Could you check a few things on this drawing? It's one solid part, dimensions in mm from its lowest x, y, z. Give positions to 0.01 mm unless a question says otherwise; leave off trailing zeros. Order: outer loops, then holes, each group sorted by start corner. A loop starts at its lowest first (then second) coordinate and runs counter-clockwise, first axis right, second up. Notation, with made-up numbers: (11.25, 9) -> (48.25, 9) arc R28 cw to (48.25, 32) -> close; hole circle Ø2 at (21.5, 51.5). An arc over 180 degrees is marked (long way). Answer as a JSON object with one key per item and string values.
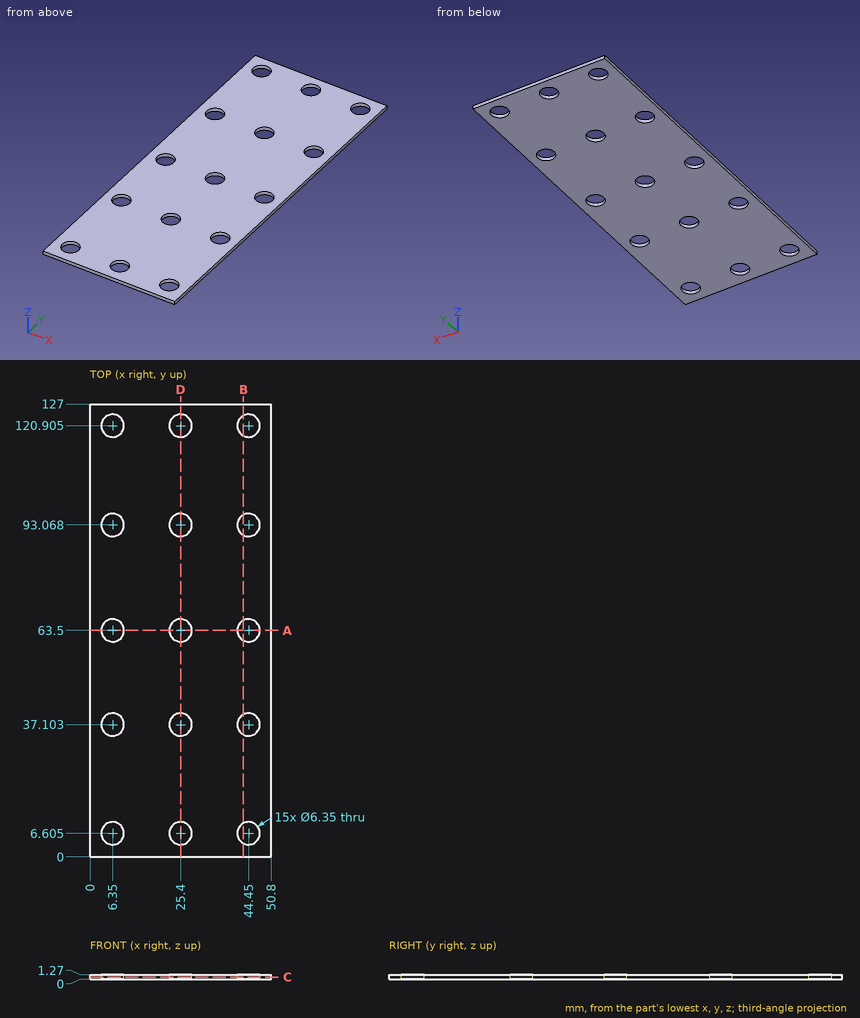
1. Will this pin go through, and if not, where does the flat tip stop? pin 1 Ø10 at (x, y) = (25.4, 120.91) entering from -Z.
Worked answers:
{"pin 1": "z = 0"}
2. If we section it at C-C on z = 0.6: Count the separate pieces of the cut face and the enclosed holes in it, then the cut area to 3 significant figures.
Worked answers:
{"separate pieces": "1", "enclosed holes": "15", "area": "5,980 mm²"}
3. Please list where these lines run through material, in increasing order: L1, parallel to X at y = 63.5, z = 0.4 (1 decimal); L2, parallel to Y at x = 44.45, z = 0.55 (1 decimal); L3, parallel to X at y = 91, z = 1.1.
Worked answers:
{"L1": "0 to 3.2, 9.5 to 22.2, 28.6 to 41.3, 47.6 to 50.8", "L2": "0 to 3.4, 9.8 to 33.9, 40.3 to 60.3, 66.7 to 89.9, 96.2 to 117.7, 124.1 to 127", "L3": "0 to 3.94, 8.76 to 22.99, 27.81 to 42.04, 46.86 to 50.8"}
4. If we section it at A-A on y = 63.5: Please give me the cut outline in (x, z) (1 decimal).
Worked answers:
{"outline": "(0, 0) -> (3.2, 0) -> (3.2, 1.3) -> (0, 1.3) -> close; (9.5, 0) -> (22.2, 0) -> (22.2, 1.3) -> (9.5, 1.3) -> close; (28.6, 0) -> (41.3, 0) -> (41.3, 1.3) -> (28.6, 1.3) -> close; (47.6, 0) -> (50.8, 0) -> (50.8, 1.3) -> (47.6, 1.3) -> close"}
5. If we section it at B-B on x = 43: Please give me the cut outline in (y, z) (1 decimal).
Worked answers:
{"outline": "(0, 0) -> (3.8, 0) -> (3.8, 1.3) -> (0, 1.3) -> close; (9.4, 0) -> (34.3, 0) -> (34.3, 1.3) -> (9.4, 1.3) -> close; (39.9, 0) -> (60.7, 0) -> (60.7, 1.3) -> (39.9, 1.3) -> close; (66.3, 0) -> (90.2, 0) -> (90.2, 1.3) -> (66.3, 1.3) -> close; (95.9, 0) -> (118.1, 0) -> (118.1, 1.3) -> (95.9, 1.3) -> close; (123.7, 0) -> (127, 0) -> (127, 1.3) -> (123.7, 1.3) -> close"}
6. If we section it at D-D on x = 25.4: Please give me the cut outline in (y, z) (1 decimal), then the cut area to 3 significant figures.
Worked answers:
{"outline": "(0, 0) -> (3.4, 0) -> (3.4, 1.3) -> (0, 1.3) -> close; (9.8, 0) -> (33.9, 0) -> (33.9, 1.3) -> (9.8, 1.3) -> close; (40.3, 0) -> (60.3, 0) -> (60.3, 1.3) -> (40.3, 1.3) -> close; (66.7, 0) -> (89.9, 0) -> (89.9, 1.3) -> (66.7, 1.3) -> close; (96.2, 0) -> (117.7, 0) -> (117.7, 1.3) -> (96.2, 1.3) -> close; (124.1, 0) -> (127, 0) -> (127, 1.3) -> (124.1, 1.3) -> close", "area": "121 mm²"}
